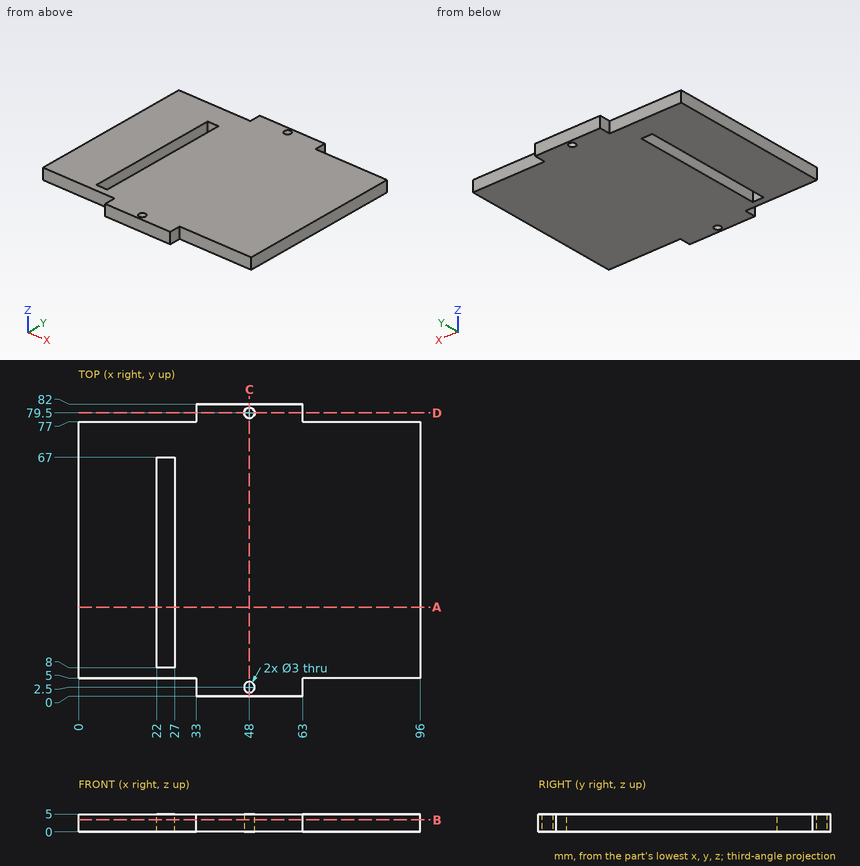
Verification items for this drawing (mm, ordinates from the low corner). Give positions to 0.01 mm unless a question says otherwise; leave off trailing zeros. Loops run counter-clockwise (first coordinate to the right, second up) from the corner with the lowest first, then second, coordinate; pieces in that order, holes last.
(1) Depth check by flat-ended pin: pin 1 Ø1.5 at (x, z) = (72.5, 3) entering from -Y; pin 2 Ø2.5 at (y, z) = (79.5, 3) entering from +X; pin 3 Ø2.5 at (x, y) = (48, 79.5) entering from +Z; pin 4 Ø2.5 at (y, z) = (3, 3) entering from -X. Enter the tip coordinate at first touch or a pass-through.
From the geometry:
pin 1: stops at y = 5
pin 2: stops at x = 63
pin 3: passes through
pin 4: stops at x = 33
(2) Section check A-A on y = 25. Record the cut outline in (x, z), then the cut area to 3 significant figures.
From the geometry:
outline: (0, 0) - (22, 0) - (22, 5) - (0, 5) - close; (27, 0) - (96, 0) - (96, 5) - (27, 5) - close
area: 455 mm2
(3) Section check D-D on y = 79.5. Record the cut outline in (x, z).
From the geometry:
outline: (33, 0) - (46.5, 0) - (46.5, 5) - (33, 5) - close; (49.5, 0) - (63, 0) - (63, 5) - (49.5, 5) - close
(4) Section check B-B on z = 3.35. Record the cut outline in (x, y), then the cut area to 3 significant figures.
From the geometry:
outline: (0, 5) - (33, 5) - (33, 0) - (63, 0) - (63, 5) - (96, 5) - (96, 77) - (63, 77) - (63, 82) - (33, 82) - (33, 77) - (0, 77) - close; hole (22, 8) - (27, 8) - (27, 67) - (22, 67) - close; hole circle Ø3 at (48, 2.5); hole circle Ø3 at (48, 79.5)
area: 6,900 mm2
(5) Section check C-C on x = 48. Record the cut outline in (y, z).
From the geometry:
outline: (0, 0) - (1, 0) - (1, 5) - (0, 5) - close; (4, 0) - (78, 0) - (78, 5) - (4, 5) - close; (81, 0) - (82, 0) - (82, 5) - (81, 5) - close
(6) Thickness scan on L1, parallel to Y at x = 48, z = 3.85; L2, parallel to X at y = 62, z = 4.4; L3, parallel to Y at x = 84, z = 2. Record the ranges inside material, lowest first.
From the geometry:
L1: y = 0 to 1, 4 to 78, 81 to 82
L2: x = 0 to 22, 27 to 96
L3: y = 5 to 77
